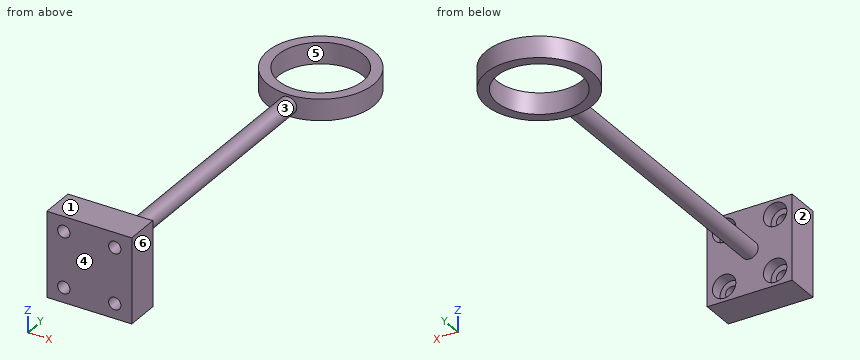
```python
from build123d import *

# Parameters (mm, degrees)
SKETCH_1_R                     = 12.5
SKETCH_1_R_2                   = 10
EXTRUDE_1_DEPTH                = 5
EXTRUDE_2_REACH                = 95.475
EXTRUDE_2_END_RADIUS           = 12.5
SKETCH_2_R                     = 2
SKETCH_3_W                     = 20
SKETCH_3_H                     = 20
EXTRUDE_3_DEPTH                = 8
HOLE_WIZARD_M2_5_1_D           = 2.9
HOLE_WIZARD_M2_5_1_CBORE_D     = 5.5
HOLE_WIZARD_M2_5_1_CBORE_DEPTH = 2.9


with BuildPart() as part:
    # 草图1 → 凸台-拉伸1 (new body)
    with BuildSketch(Plane.XY):
        Circle(SKETCH_1_R)
        Circle(SKETCH_1_R_2, mode=Mode.SUBTRACT)
    extrude(amount=EXTRUDE_1_DEPTH)

    # 凸台-拉伸2: up to this cylinder (the profile starts outside it)
    extrude_2_end = Plane(origin=(0, 0, 2.5), z_dir=(0, 0, -1)) * Cylinder(EXTRUDE_2_END_RADIUS, 216.95, mode=Mode.PRIVATE)
    # 草图2 → 凸台-拉伸2 (add, up to the surface)
    with BuildSketch(Plane(origin=(0, -80, 0), x_dir=(1, 0, 0), z_dir=(0, 1, 0)), mode=Mode.PRIVATE) as extrude_2_sk1:
        with Locations(Location((0, -2.5, 0), (0, 0, 90))):
            Circle(SKETCH_2_R)
    extrude_2_tool1 = extrude(extrude_2_sk1.sketch, amount=EXTRUDE_2_REACH, mode=Mode.PRIVATE) - extrude_2_end
    add(extrude_2_tool1.solids().sort_by_distance((0, -80, 2.5))[0])

    # 草图3 → 凸台-拉伸3 (add)
    with BuildSketch(Plane.XZ.offset(80)):
        with Locations((0, 2.5)):
            Rectangle(SKETCH_3_W, SKETCH_3_H)
    extrude(amount=EXTRUDE_3_DEPTH)

    # M2.5 六角凹头螺钉的柱形沉头孔1 (through all)
    with Locations(Plane(origin=(0, -80, 0), x_dir=(1, 0, 0), z_dir=(0, 1, 0))):
        with Locations((-6, 4), (6, 4), (6, -9), (-6, -9)):
            CounterBoreHole(HOLE_WIZARD_M2_5_1_D / 2, HOLE_WIZARD_M2_5_1_CBORE_D / 2, HOLE_WIZARD_M2_5_1_CBORE_DEPTH)


solid = part.part
```
Work out the finished part from the listing and answer in its coordinate system (mm). Face numbers are marked on the shaded views. A direction names the side the tool comes from. Round coordinates to 2 decimals unless told otherwise and drop trailing zeros. Write each loop counter-clockwise with the first axis right and the second up, starting at its lowest first coordinate (ties: lowest second). Pieces come first, ordered by that corner, then holes. Notation, with made-up numbers: (-27.75, 21.25) -> (16.25, 21.25) arc R20 ccw to (16.25, 50.25) -> close; hole circle Ø3 at (20.25, 87.25). An arc over 180 degrees is marked (long way). Write each question's results on one line, items separated by ' | '.
Q1. Section A-A, the plane x = 0 is taken. Write down the section's boundary in (y, z), then the cut area to 3 significant figures.
Data:
outline: (-88, -7.5) -> (-80, -7.5) -> (-80, 0.5) -> (-12.5, 0.5) -> (-12.5, 0) -> (-10, 0) -> (-10, 5) -> (-12.5, 5) -> (-12.5, 4.5) -> (-80, 4.5) -> (-80, 12.5) -> (-88, 12.5) -> close; (10, 0) -> (12.5, 0) -> (12.5, 5) -> (10, 5) -> close | area: 455 mm^2
Q2. Section C-C, the plane y = 0 is taken. Write down the section's boundary in (x, z), then the cut area to 3 significant figures.
Data:
outline: (-12.5, 0) -> (-10, 0) -> (-10, 5) -> (-12.5, 5) -> close; (10, 0) -> (12.5, 0) -> (12.5, 5) -> (10, 5) -> close | area: 25.0 mm^2
Q3. Section D-D, the plane x = -6 is taken. Write down the section's boundary in (y, z).
Data:
outline: (-88, -7.5) -> (-80, -7.5) -> (-80, -6.75) -> (-82.9, -6.75) -> (-82.9, -5.45) -> (-88, -5.45) -> close; (-88, -2.55) -> (-82.9, -2.55) -> (-82.9, -1.25) -> (-80, -1.25) -> (-80, 6.25) -> (-82.9, 6.25) -> (-82.9, 7.55) -> (-88, 7.55) -> close; (-88, 10.45) -> (-82.9, 10.45) -> (-82.9, 11.75) -> (-80, 11.75) -> (-80, 12.5) -> (-88, 12.5) -> close; (-10.97, 0) -> (-8, 0) -> (-8, 5) -> (-10.97, 5) -> close; (8, 0) -> (10.97, 0) -> (10.97, 5) -> (8, 5) -> close
Q4. Straight lines are drawn through the part: line 1 along Z through (x, y) = (-6, -84.35); line 2 along Z through (x, y) = (6, -81.25); line 3 along X through (y, z) = (-80.5, 11.5). For each, find the intervals that lie inside material, in ascending order. Write a range as [from, to].
Data:
line 1: [-7.5, -5.45], [-2.55, 7.55], [10.45, 12.5] | line 2: [-7.5, -6.75], [-1.25, 6.25], [11.75, 12.5] | line 3: [-10, -7.15], [-4.85, 4.85], [7.15, 10]
Q5. Section B-B, the plane z = 2.5 is taken. Write down the section's boundary in (x, y), then the cut area to 3 significant figures.
Data:
outline: (-10, -88) -> (10, -88) -> (10, -80) -> (2, -80) -> (2, -12.34) arc R12.5 ccw (long way) to (-2, -12.34) -> (-2, -80) -> (-10, -80) -> close; hole circle Ø20 at (0, 0) | area: 607 mm^2
Q6. Determine the mould class of the marked faces 4, 5 and 6 for opening direction Y: released by +Y, released by -Y, zero draft, split by the parting line, or undercut.
Data:
face 4: released by -Y | face 5: undercut | face 6: zero draft
Q7. Which of the six approach directions +Z, -Z, +X, -X, +Y, -Y give full straight-line access (tool end or side, diameter ignored) to the marked faces 1, 2 and 3?
Data:
face 1: +Z, +X, -X, +Y, -Y | face 2: +Z, -Z, -X, -Y | face 3: none
Q8. Flat-ended cylindrical pins translate along their axes: P1, Ø9, axis at x = -6, z = 9, coming from the -Y side; P2, Ø8, axis at x = -8.5, z = 8, coming from the +Y side; P3, Ø3.5, axis at x = 6, z = -4, coming from the +Y side; P4, Ø12.5, axis at x = 4, y = 6, coming from the +Z side. Find the tip coordinate at first contact, or state that the pin passes through.
Data:
P1: y = -88 | P2: y = 11.04 | P3: y = -82.9 | P4: z = 5
